from build123d import *

# Parameters (mm, degrees)
SKETCH_W     = 110
SKETCH_H     = 110
PAD_DEPTH    = 3
SKETCH001_R  = 5
PAD001_DEPTH = 10


with BuildPart() as part:
    # Sketch → Pad (new body)
    with BuildSketch(Plane.XY):
        Rectangle(SKETCH_W, SKETCH_H)
    extrude(amount=PAD_DEPTH)

    # Sketch001 (on Face6 of Pad) → Pad001 (join)
    with BuildSketch(Plane.XY.offset(3)):
        with Locations((-45, 45)):
            Circle(SKETCH001_R)
        with Locations((45, 45)):
            Circle(SKETCH001_R)
        with Locations((45, -45)):
            Circle(SKETCH001_R)
        with Locations((-45, -45)):
            Circle(SKETCH001_R)
        with Locations((-35, 45)):
            Circle(SKETCH001_R)
        with Locations((-25, 45)):
            Circle(SKETCH001_R)
        with Locations((-45, 35)):
            Circle(SKETCH001_R)
        with Locations((35, 45)):
            Circle(SKETCH001_R)
        with Locations((25, 45)):
            Circle(SKETCH001_R)
        with Locations((-45, -35)):
            Circle(SKETCH001_R)
        with Locations((-35, -45)):
            Circle(SKETCH001_R)
        with Locations((-25, -45)):
            Circle(SKETCH001_R)
        with Locations((35, -45)):
            Circle(SKETCH001_R)
        with Locations((25, -45)):
            Circle(SKETCH001_R)
    extrude(amount=PAD001_DEPTH)


solid = part.part
Input: part model. Units: mm. Frame: model coordinates. A direction names the side the tool comes from. Coordinates: 2 decimals unless noted, no trailing zeros. Order: outer loops, then holes, each group sorted by start corner. A loop starts at its lowest first (then second) coordinate and runs counter-clockwise, first axis right, second up. Notation, with made-up numbers: M -36,1.5 L 16,1.5 A18 cw 16,35.5 Z; hole C -13,26.5 d7. An arc over 180 degrees is marked long. Write item = value, one per line. Start each with the question number.
(1) Section B-B on x = 45. Output: boundary loops of the cut face in (y, z).
(2) Pull-direction query (X, two-part tool) for faces 3 (the cylindrical face through (49, -48, 8)), 4 (the cylindrical face through (35, -50, 8)), 5 (the flat face through (35, -45, 13)); classes: released by +X, released by -X, zero draft, split by the parting line, or undercut.
(3) First-contact query: P1, Ø12, axis at x = -1.5, y = -15.5, coming from the +Z side. Flat tip, straight axial feed; report the tip coordinate or a pass-through.
(4) Section C-C on y = 42.5. Output: boundary loops of the cut face in (x, z).
(5) Section D-D on x = 11. Output: boundary loops of the cut face in (y, z).
(6) Reachability of faces 1 (the flat face through (-1, -55, 1)), 2 (the flat face through (-1, 1, 3)) from +Z, -Z, +X, -X, +Y, -Y: full face, straight path, thin tool, end or side. Return the list, or none.
(7) Line query: line 1 along Y through (x, z) = (-25, 10); line 2 along X through (y, z) = (-46, 7); line 3 along Z through (x, y) = (25.5, 17.5). Output: solid intervals per line, ascending. Write a range as [from, to].
Result set:
q1.outline = M -55,0 L 55,0 L 55,3 L 50,3 L 50,13 L 40,13 L 40,3 L -40,3 L -40,13 L -50,13 L -50,3 L -55,3 Z
q2.face_3 = undercut
q2.face_4 = undercut
q2.face_5 = zero draft
q3.P1 = 3
q4.outline = M -55,0 L 55,0 L 55,3 L 49.33,3 L 49.33,13 L 40.67,13 L 40.67,3 L 39.33,3 L 39.33,13 L 30.67,13 L 30.67,3 L 29.33,3 L 29.33,13 L 20.67,13 L 20.67,3 L -20.67,3 L -20.67,13 L -29.33,13 L -29.33,3 L -30.67,3 L -30.67,13 L -39.33,13 L -39.33,3 L -40.67,3 L -40.67,13 L -49.33,13 L -49.33,3 L -55,3 Z
q5.outline = M -55,0 L 55,0 L 55,3 L -55,3 Z
q6.face_1 = +Z, -Z, +X, -X, -Y
q6.face_2 = +Z
q7.line_1 = [-50, -40], [40, 50]
q7.line_2 = [-49.9, -40.1], [-39.9, -30.1], [-29.9, -20.1], [20.1, 29.9], [30.1, 39.9], [40.1, 49.9]
q7.line_3 = [0, 3]
